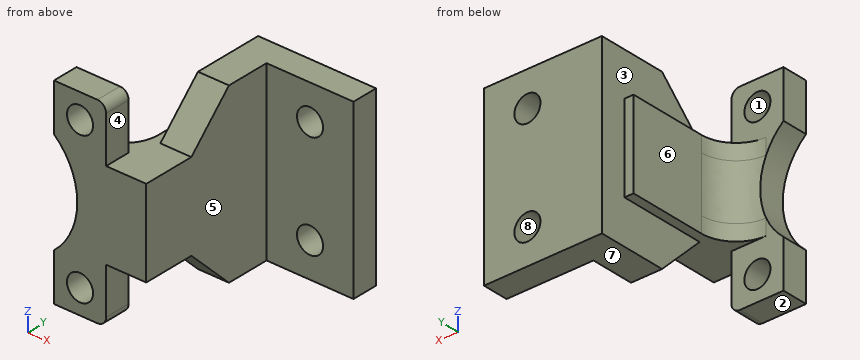
from build123d import *

# Parameters (mm, degrees)
SKETCH1_R           = 1.5
BOSS_EXTRUDE1_DEPTH = 3
SKETCH3_W           = 4.615398666
SKETCH3_H           = 10
BOSS_EXTRUDE2_DEPTH = 12.9997796
FILLET7_R           = 1
CUT_EXTRUDE4_DEPTH  = 10
SKETCH9_W           = 13.564457496
SKETCH9_H           = 20
SKETCH9_R           = 1.5
BOSS_EXTRUDE3_DEPTH = 3
CHAMFER1_SIZE       = 10
CHAMFER2_SIZE       = 10
FILLET8_R           = 4


with BuildPart() as part:
    # Sketch1 → Boss-Extrude1 (new body)
    with BuildSketch(Plane(origin=(0, 0, 0), x_dir=(1, 0, 0), z_dir=(0, 1, 0))):
        Polygon((-3, -11.32792047), (3, -11.32792047), (3, -5), (7.615398666, -5), (7.615398666, 5), (3, 5), (3, 11.32792047), (-3, 11.32792047), align=None)
        with Locations(Location((0, 8.5, 0), (0, 0, 270))):
            Circle(SKETCH1_R, mode=Mode.SUBTRACT)
        with Locations(Location((0, -8.5, 0), (0, 0, 270))):
            Circle(SKETCH1_R, mode=Mode.SUBTRACT)
    extrude(amount=BOSS_EXTRUDE1_DEPTH)

    # Sketch3 → Boss-Extrude2 (add)
    with BuildSketch(Plane(origin=(0, 3, 0), x_dir=(1, 0, 0), z_dir=(0, 1, 0))):
        with Locations((5.307699333, 0)):
            Rectangle(SKETCH3_W, SKETCH3_H)
    extrude(amount=BOSS_EXTRUDE2_DEPTH)

    # Fillet7
    fillet7_edges = [part.edges().sort_by_distance(p)[0] for p in [
        (3, 1.5, 11.32792047),
        (3, 1.5, -11.32792047),
    ]]
    fillet(fillet7_edges, radius=FILLET7_R)

    # Sketch7 → Cut-Extrude4 (cut)
    with BuildSketch(Plane.XZ):
        with BuildLine():
            Line((-3.65526474, -6.392053518), (-3.78188192, 6.478485425))
            ThreePointArc((-3.78188192, 6.478485425), (-0.319780446, 0.076652438), (-3.65526474, -6.392053518))
        make_face()
    extrude(amount=-CUT_EXTRUDE4_DEPTH, mode=Mode.SUBTRACT)

    # Sketch9 → Boss-Extrude3 (add)
    with BuildSketch(Plane(origin=(0, 15.9997796, 0), x_dir=(1, 0, 0), z_dir=(0, 1, 0))):
        with Locations((10.833169918, 0)):
            Rectangle(SKETCH9_W, SKETCH9_H)
        with Locations(Location((12.615398666, 6, 0), (0, 0, 270))):
            Circle(SKETCH9_R, mode=Mode.SUBTRACT)
        with Locations(Location((12.615398666, -6, 0), (0, 0, 270))):
            Circle(SKETCH9_R, mode=Mode.SUBTRACT)
    extrude(amount=BOSS_EXTRUDE3_DEPTH)

    # Chamfer1
    # the kernel refuses this chamfer: 10 mm, written as the material it adds along each edge
    with BuildSketch(Plane(origin=(4.05094117, 15.9997796, 5), x_dir=(0, -0.9996219169112968, -0.027495876610586403), z_dir=(1, 0, 0))) as chamfer1_piece_1_section:
        Polygon((CHAMFER1_SIZE * 0.999621916911, -CHAMFER1_SIZE * 0.0274958766106), (-CHAMFER1_SIZE * 0.0274958766106, -CHAMFER1_SIZE * 0.999621916911), (0, 0), align=None)
    chamfer1_piece_1 = extrude(amount=3.564457497, mode=Mode.PRIVATE)
    chamfer1_piece_1 = split(chamfer1_piece_1, bisect_by=Plane(origin=(5.833169918, 12.110890711, 10), z_dir=(0, 0, -1)), keep=Keep.TOP, mode=Mode.PRIVATE)
    add(chamfer1_piece_1)

    # Chamfer2
    # the kernel refuses this chamfer: 10 mm, written as the material it adds along each edge
    with BuildSketch(Plane(origin=(7.615398666, 15.9997796, -5), x_dir=(0, -0.9996219169112968, 0.027495876610586403), z_dir=(-1, 0, 0))) as chamfer2_piece_1_section:
        Polygon((CHAMFER2_SIZE * 0.999621916911, -CHAMFER2_SIZE * 0.0274958766106), (-CHAMFER2_SIZE * 0.0274958766106, -CHAMFER2_SIZE * 0.999621916911), (0, 0), align=None)
    chamfer2_piece_1 = extrude(amount=3.564457497, mode=Mode.PRIVATE)
    chamfer2_piece_1 = split(chamfer2_piece_1, bisect_by=Plane(origin=(5.833169918, 12.110890711, -10), z_dir=(0, 0, 1)), keep=Keep.TOP, mode=Mode.PRIVATE)
    add(chamfer2_piece_1)

    # Fillet8
    fillet8_edges = [part.edges().sort_by_distance(p)[0] for p in [
        (3, 3, 0),
    ]]
    fillet(fillet8_edges, radius=FILLET8_R)


solid = part.part
Work out the finished part from the listing and answer in its coordinate system (mm). Face numbers are marked on the shaded views. A direction names the side the tool comes from. Round coordinates to 2 decimals unless told otherwise and drop trailing zeros. Write each loop counter-clockwise with the first axis right and the second up, starting at its lowest first coordinate (ties: lowest second). Pieces come first, ordered by that corner, then holes. Notation, with made-up numbers: (48, 76) - (79, 76) arc R22 ccw to (79, 100) - close; hole circle Ø9 at (66.25, 17). An arc over 180 degrees is marked (long way). Answer in a Markdown table with one row per item. Add a question column.
1. A cutting plane is placed at C-C, the plane x = 9. Determine the outline of the cut face in (y, z), and give its area (3 significant figures).
2. A cutting plane is placed at D-D, the plane y = 9.25. Determine the outline of the cut face in (x, z), and give its area (3 significant figures).
3. Given pin 1 (2 mm diameter, centred on y = 8, z = 8.5, fed in from +X); pin 2 (5 mm diameter, centred on x = 14.5, z = 2.5, fed in from -Y); pin 3 (5 mm diameter, centred on x = 1, z = -6, fed in from +Y); pin 4 (1.5 mm diameter, centred on y = 2, z = -6.5, fed in from +X), each flat-ended and moving along its own axis, determine where each tip first touches the part or whether it passes through.
4. The mould has two halves that part along Z. Classify the marked faces 6, 7 and 8: +Z half, -Z half, draft (parallel to the pull), parting line (faces both ways), or undercut.
5. A cutting plane is placed at B-B, the plane y = 13.25. Determine the outline of the cut face in (x, z), and give its area (3 significant figures).
6. Find the intervals of material crossed by line 1 along X through (y, z) = (1.75, -8.5); line 2 along X through (y, z) = (17.15, -6); line 3 along X through (y, z) = (7.5, -0.25), in increasing order. Write a range as from..to.
7. A cutting plane is placed at A-A, the plane z = 8.5. Determine the outline of the cut face in (x, y), and give its area (3 significant figures).
8. For the marked faces 1, 2, 3, 4 and 5, determine the directions among +Z, -Z, +X, -X, +Y, -Y from which every point of the face is accessible in a straight line to the end or side of a thin tool.
Worked out:
| question | item | result |
|---|---|---|
| 1 | outline | (16, -10) - (19, -10) - (19, 10) - (16, 10) - close |
| 1 | area | 60.0 mm^2 |
| 2 | outline | (3, -5) - (4.05, -5) - (4.05, -8.25) - (7.62, -8.25) - (7.62, 8.25) - (4.05, 8.25) - (4.05, 5) - (3, 5) - close |
| 2 | area | 69.3 mm^2 |
| 3 | pin 1 | through |
| 3 | pin 2 | y = 16 |
| 3 | pin 3 | y = 16 |
| 3 | pin 4 | x = 3 |
| 4 | face 6 | draft |
| 4 | face 7 | -Z half |
| 4 | face 8 | undercut |
| 5 | outline | (3, -5) - (4.05, -5) - (4.05, -10) - (7.62, -10) - (7.62, 10) - (4.05, 10) - (4.05, 5) - (3, 5) - close |
| 5 | area | 81.8 mm^2 |
| 6 | line 1 | -3..-1.5, 1.5..3 |
| 6 | line 2 | 4.05..11.12, 14.12..17.62 |
| 6 | line 3 | 3..7.62 |
| 7 | outline | (-3, 0) - (-1.5, 0) - (-1.5, 3) - (-3, 3) - close; (1.5, 0) - (3, 0) - (3, 3) - (1.5, 3) - close; (4.05, 9.5) - (7.62, 9.5) - (7.62, 16) - (17.62, 16) - (17.62, 19) - (4.05, 19) - close |
| 7 | area | 72.9 mm^2 |
| 8 | face 1 | +Y, -Y |
| 8 | face 2 | -Z, +X, -X, +Y, -Y |
| 8 | face 3 | -X, +Y |
| 8 | face 4 | +Z, +X, +Y, -Y |
| 8 | face 5 | +Z, -Z, +X, -Y |
